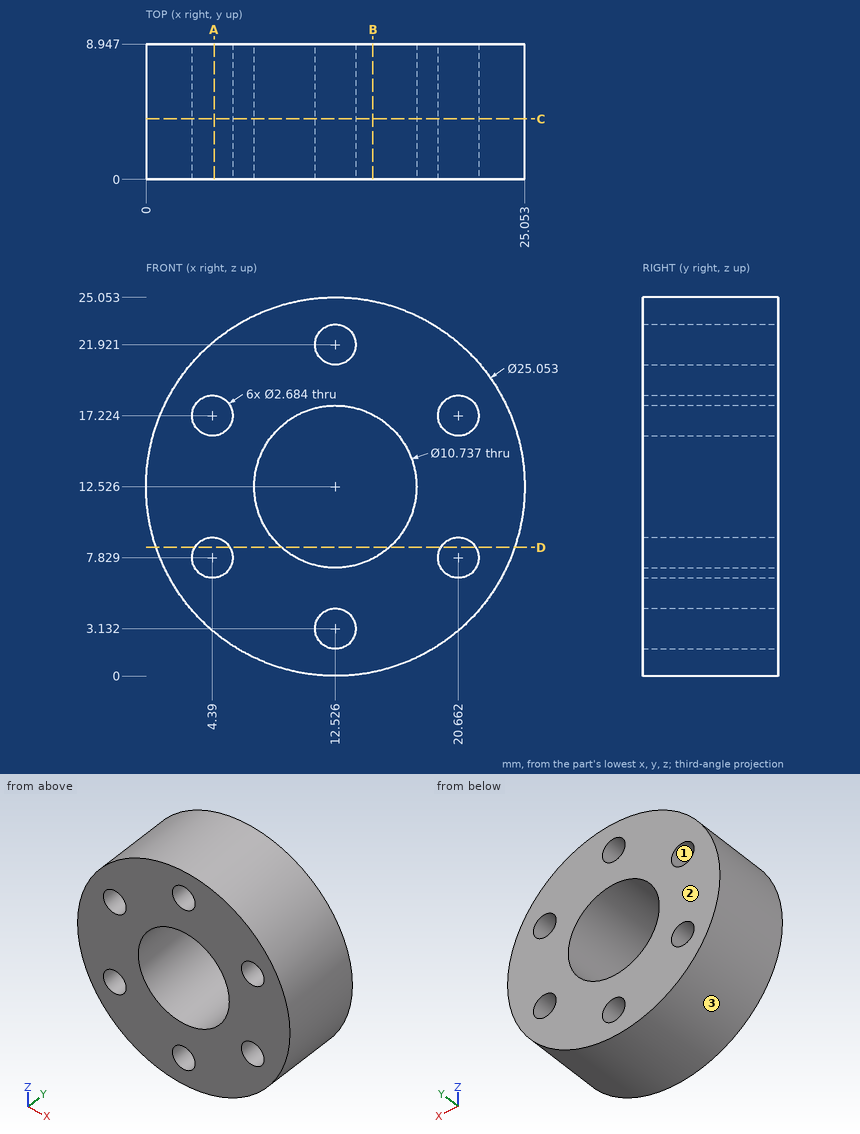
Drawing for the job (mm, zero at the part's lowest x, y, z). Round coordinates to 2 decimals unless told otherwise and drop trailing zeros. Write each loop counter-clockwise with the first axis right and the second up, starting at its lowest first coordinate (ties: lowest second). Pieces come first, ordered by that corner, then holes. Notation, with made-up numbers: M -27.5,25 L 4.5,25 A18 cw 4.5,52 Z; hole C 87.25,51 d10. An arc over 180 degrees is marked long. Answer as a JSON object with one key per item and string values. Group by question number.
(1) Cut at B-B (x = 15). Give the cut face in (y, z).
(2) Cut at C-C (y = 4). Give the cut face in (x, z) (1 decimal).
(3) Cut at D-D (z = 8.5). Give the cut face in (x, y) (1 decimal), and give its area (3 significant figures).
(4) Mould opens along X. For the marked faces 1, 2 and 3 say: pulls with the +X half, pulls with the -X half, needs draft (parallel to the pull), parting line crosses it, or undercut.
(5) Drill centre lines: L1, parallel to Z at x = 12.5, y = 0.75 (1 decimal); L2, parallel to X at y = 4.5, z = 18 (1 decimal); L3, parallel to X at y = 5.5, z = 6.75 (1 decimal). Where is each one in solid material? Low to high.
(6) Cut at A-A (x = 4.5). Give the cut face in (y, z).
(7) Flat gauge pins, fed straight in: pin 1 (4.5 mm diameter, centred on x = 20.66, z = 17.22, fed in from +Y); pin 2 (1.5 mm diameter, centred on x = 5.5, y = 1, fed in from +Z); pin 3 (1.5 mm diameter, centred on x = 17, y = 4.5, fed in from -Z); pin 4 (5 mm diameter, centred on x = 8, y = 7.5, fed in from -Z) (1 decimal). Where does each tip first touch, or does it go through?
Responses:
{
 "1": {"outline": "M 0,0.25 L 8.95,0.25 L 8.95,7.76 L 0,7.76 Z; M 0,17.29 L 8.95,17.29 L 8.95,24.81 L 0,24.81 Z"},
 "2": {"outline": "C 12.5,12.5 d25.1; hole C 4.4,7.8 d2.7; hole C 4.4,17.2 d2.7; hole C 12.5,12.5 d10.7; hole C 12.5,3.1 d2.7; hole C 12.5,21.9 d2.7; hole C 20.7,7.8 d2.7; hole C 20.7,17.2 d2.7"},
 "3": {"outline": "M 0.7,0 L 3.2,0 L 3.2,8.9 L 0.7,8.9 Z; M 5.6,0 L 9,0 L 9,8.9 L 5.6,8.9 Z; M 16.1,0 L 19.5,0 L 19.5,8.9 L 16.1,8.9 Z; M 21.8,0 L 24.4,0 L 24.4,8.9 L 21.8,8.9 Z", "area": "107 mm2"},
 "4": {"face 1": "undercut", "face 2": "needs draft", "face 3": "parting line crosses it"},
 "5": {"L1": "z = 0 to 1.8, 4.5 to 7.2, 17.9 to 20.6, 23.3 to 25.1", "L2": "x = 1.3 to 3.3, 5.5 to 19.6, 21.8 to 23.8", "L3": "x = 1.4 to 3.6, 5.2 to 19.9, 21.5 to 23.6"},
 "6": {"outline": "M 0,2.91 L 8.95,2.91 L 8.95,6.49 L 0,6.49 Z; M 0,9.17 L 8.95,9.17 L 8.95,15.89 L 0,15.89 Z; M 0,18.56 L 8.95,18.56 L 8.95,22.14 L 0,22.14 Z"},
 "7": {"pin 1": "stops at y = 8.95", "pin 2": "stops at z = 23.37", "pin 3": "stops at z = 0.57", "pin 4": "stops at z = 0.2"}
}
